```python
from build123d import *

# Parameters (mm, degrees)
F5_W      = 180
F5_H      = 140
F0_DEPTH  = 5
F1_R      = 2
F7_DEPTH  = 8
F8_W      = 75
F8_H      = 10
F8_W_2    = 80
F9_DEPTH  = 75
F10_DEPTH = 75
F11_DEPTH = 25
F4_DEPTH  = 25
F12_R     = 1.5


with BuildPart() as f0:
    # F5 (on Top) → F0 (new body)
    with BuildSketch(Plane.XY):
        with Locations((5.4015538096, 34.1141599765)):
            Rectangle(F5_W, F5_H)
    extrude(amount=F0_DEPTH)

    # F1
    f1_edges = [f0.edges().sort_by_distance(p)[0] for p in [
        (5.401554, -35.88584, 5),
        (95.401554, 34.11416, 5),
        (-84.598446, 34.11416, 5),
        (5.401554, 104.11416, 5),
    ]]
    fillet(f1_edges, radius=F1_R)

    # F6 (on face) → F7 (join)
    with BuildSketch(Plane.XY.offset(5)):
        with BuildLine():
            ThreePointArc((82.8569015917, 15.7776214182), (53.4015538096, 37.1141599765), (23.9462060275, 15.7776214182))
            Line((23.9462060275, 15.7776214182), (34.0379001592, 15.7776214182))
            ThreePointArc((34.0379001592, 15.7776214182), (53.4015538096, 27.7551758891), (72.7652074601, 15.7776214182))
            Line((72.7652074601, 15.7776214182), (82.8569015917, 15.7776214182))
        make_face()
    extrude(amount=F7_DEPTH)

    # F8 (on face) → F9 (join)
    with BuildSketch(Plane.XY.offset(5)):
        with Locations((-38.0984461904, 87.1141599765)):
            Rectangle(F8_W, F8_H)
        with Locations((46.4015538096, 57.1141599765)):
            Rectangle(F8_W_2, F8_H)
    extrude(amount=F9_DEPTH)

    # F8 (on face) → F10 (join)
    with BuildSketch(Plane.XY.offset(5)):
        with Locations((-38.0984461904, 87.1141599765)):
            Rectangle(F8_W, F8_H)
        with Locations((46.4015538096, 57.1141599765)):
            Rectangle(F8_W_2, F8_H)
    extrude(amount=F10_DEPTH)

    # F2 (on face) → F11 (cut)
    with BuildSketch(Plane.XZ.offset(-52.1141599765)):
        with BuildLine():
            Line((13.9015538096, 80), (13.9015538096, 67.5))
            ThreePointArc((13.9015538096, 67.5), (46.4015538096, 35), (78.9015538096, 67.5))
            Line((78.9015538096, 67.5), (78.9015538096, 80))
            Line((78.9015538096, 80), (13.9015538096, 80))
        make_face()
    extrude(amount=-F11_DEPTH, mode=Mode.SUBTRACT)

    # F3 (on face) → F4 (cut)
    with BuildSketch(Plane.XZ.offset(-82.1141599765)):
        with BuildLine():
            Line((-68.0984461904, 70), (-68.0984461904, 55))
            ThreePointArc((-68.0984461904, 55), (-38.0984461904, 25), (-8.0984461904, 55))
            Line((-8.0984461904, 55), (-8.0984461904, 70))
            Line((-8.0984461904, 70), (-0.5984461904, 70))
            Line((-0.5984461904, 70), (-0.5984461904, 80))
            Line((-0.5984461904, 80), (-75.5984461904, 80))
            Line((-75.5984461904, 80), (-75.5984461904, 70))
            Line((-75.5984461904, 70), (-68.0984461904, 70))
        make_face()
    extrude(amount=-F4_DEPTH, mode=Mode.SUBTRACT)

    # F12
    f12_edges = [f0.edges().sort_by_distance(p)[0] for p in [
        (86.401554, 52.11416, 42.5),
        (86.401554, 62.11416, 42.5),
        (78.901554, 57.11416, 80),
        (13.901554, 57.11416, 80),
        (-8.098446, 87.11416, 70),
        (-68.098446, 87.11416, 70),
        (6.401554, 52.11416, 42.5),
        (6.401554, 62.11416, 42.5),
        (-75.598446, 82.11416, 37.5),
        (-75.598446, 92.11416, 37.5),
        (-0.598446, 82.11416, 37.5),
        (-0.598446, 92.11416, 37.5),
        (86.401554, 57.11416, 80),
        (6.401554, 57.11416, 80),
        (-0.598446, 87.11416, 70),
        (-75.598446, 87.11416, 70),
        (10.151554, 52.11416, 80),
        (-4.348446, 82.11416, 70),
        (-71.848446, 92.11416, 70),
        (-4.348446, 92.11416, 70),
        (-71.848446, 82.11416, 70),
        (10.151554, 62.11416, 80),
        (82.651554, 52.11416, 80),
        (46.401554, 52.11416, 35),
        (-38.098446, 82.11416, 25),
        (82.651554, 62.11416, 80),
        (46.401554, 62.11416, 35),
        (-38.098446, 92.11416, 25),
        (53.401554, 27.755176, 13),
        (28.992053, 15.777621, 13),
        (77.811055, 15.777621, 13),
    ]]
    fillet(f12_edges, radius=F12_R)


solid = f0.part
```
Build history of the part. All positions in model axes, mm. A direction names the side the tool comes from. Give positions to 0.01 mm unless a question says otherwise; leave off trailing zeros. Loops run counter-clockwise (first coordinate to the right, second up) from the corner with the lowest first, then second, coordinate; pieces in that order, holes last.
1) Probe line 1 along Z through (x, y) = (62, 29.5); line 2 along Y through (x, z) = (-2.5, 48.5); line 3 along Y through (x, z) = (76.5, 28). List the from-to ranges inside material, lowest first.
Values follow:
line 1: z = 0 to 13
line 2: y = 82.11 to 92.11
line 3: y = 52.11 to 62.11
2) Band-saw the part on C-C on z = 43.5. State how many separate pieces and enclosed holes the cut face has, then the cut area to 3 significant figures.
Values follow:
separate pieces: 4
enclosed holes: 0
area: 549 mm2
3) Drop flat-ended pins along their axis: P1, Ø3, axis at x = 77, z = 8, coming from the -Y side; P2, Ø5, axis at x = -52.5, z = 32, coming from the -Y side; P3, Ø5, axis at x = -4, y = 87, coming from the +Z side; P4, Ø3.5, axis at y = 88, z = 59, coming from the +X side. Give the stop position or say it passes through.
Values follow:
P1: stops at y = 15.78
P2: passes through
P3: stops at z = 70
P4: stops at x = -0.6
4) Two-plate mould, pull along X, no slides. Class faces 1 (the face through (-75.598, 87, 36)), 2 (the face through (13.902, 57, 73)), 3 (the face through (86.402, 57, 41)): released by +X, released by -X, zero draft, split by the parting line, or undercut.
Values follow:
face 1: released by -X
face 2: undercut
face 3: released by +X
5) 3-axis set-ups, long thin cutter, end or side, ignore diameter. For faces 4 (the face through (-8.098, 87, 62)), 5 (the face through (-39, 82.114, 22)), 6 (the face through (6.402, 57, 41)): which of +Z, -Z, +X, -X, +Y, -Y reach the whole face in a straight line?
Values follow:
face 4: +Z, +Y, -Y
face 5: +Z, +X, -X, -Y
face 6: +Z, -X, +Y, -Y
6) Band-saw the part on B-B on y = 44.5. List the corners of the cut face in (x, z), then the cut area to 3 significant figures.
Values follow:
outline: (-84.6, 0) - (95.4, 0) - (95.4, 3) arc R2 ccw to (93.4, 5) - (-82.6, 5) arc R2 ccw to (-84.6, 3) - close
area: 898 mm2
7) Band-saw the part on A-A on z = 73.5. List the corners of the cut face in (x, y), then the cut area to 3 significant figures.
Values follow:
outline: (6.4, 53.61) arc R1.5 ccw to (7.9, 52.11) - (12.4, 52.11) arc R1.5 ccw to (13.9, 53.61) - (13.9, 60.61) arc R1.5 ccw to (12.4, 62.11) - (7.9, 62.11) arc R1.5 ccw to (6.4, 60.61) - close; (78.9, 53.61) arc R1.5 ccw to (80.4, 52.11) - (84.9, 52.11) arc R1.5 ccw to (86.4, 53.61) - (86.4, 60.61) arc R1.5 ccw to (84.9, 62.11) - (80.4, 62.11) arc R1.5 ccw to (78.9, 60.61) - close
area: 146 mm2
